from build123d import *

# Parameters (mm, degrees)
SKETCH1_W                                         = 25.4
SKETCH1_H                                         = 6
SKETCH2_R                                         = 15
BOSS_EXTRUDE1_DEPTH                               = 55.54
CUT_EXTRUDE1_DEPTH                                = 62.54
SKETCH4_W                                         = 7.0104
SKETCH4_H                                         = 61.54
F_2_CLEARANCE_HOLE1_D                             = 2.5
F_2_CLEARANCE_HOLE1_DEPTH                         = 12
SKETCH7_W                                         = 1.25
SKETCH7_H                                         = 16.341500105
CSK_FOR_8_FLAT_HEAD_MACHINE_SCREW_100_D           = 4.5
CSK_FOR_8_FLAT_HEAD_MACHINE_SCREW_100_DEPTH       = 61.54
CSK_FOR_8_FLAT_HEAD_MACHINE_SCREW_100_CSINK_D     = 9.4
CSK_FOR_8_FLAT_HEAD_MACHINE_SCREW_100_CSINK_ANGLE = 90
SKETCH11_R                                        = 10.3124
CUT_EXTRUDE2_DEPTH                                = 38.1


with BuildPart() as part:
    # Sketch1 → Revolve1 (revolve)
    with BuildSketch(Plane.XZ):
        with Locations((12.7, 58.54)):
            Rectangle(SKETCH1_W, SKETCH1_H)
    revolve(axis=Axis((0, 0, 61.54), (0, 0, -1)))

    # Sketch2 → Boss-Extrude1 (add)
    with BuildSketch(Plane(origin=(0, 0, 55.54), x_dir=(-1, 0, 0), z_dir=(0, 0, -1))):
        Circle(SKETCH2_R)
    extrude(amount=BOSS_EXTRUDE1_DEPTH)

    # Sketch3 → Cut-Extrude1 (cut, through all)
    with BuildSketch(Plane(origin=(0, 0, 0), x_dir=(-1, 0, 0), z_dir=(0, 0, -1))):
        with BuildLine():
            Line((2.5, 9.058499895), (-2.5, 9.058499895))
            Line((-2.5, 9.058499895), (-2.5, 6.538348415))
            ThreePointArc((-2.5, 6.538348415), (0, 7), (2.5, 6.538348415))
            Line((2.5, 6.538348415), (2.5, 9.058499895))
        make_face()
    extrude(amount=-CUT_EXTRUDE1_DEPTH, mode=Mode.SUBTRACT)

    # Sketch4 → Cut-Revolve1 (revolve, cut)
    with BuildSketch(Plane.XZ):
        with Locations((3.5052, 30.77)):
            Rectangle(SKETCH4_W, SKETCH4_H)
    revolve(axis=Axis((0, 0, 61.54), (0, 0, -1)), mode=Mode.SUBTRACT)

    # #2 Clearance Hole1
    with Locations(Plane(origin=(0, 0, 0), x_dir=(-1, 0, 0), z_dir=(0, 0, -1))):
        with Locations((-11.5, 0), (-5.75, -9.959292144), (5.75, -9.959292144), (11.5, 0), (5.75, 9.959292144), (-5.75, 9.959292144)):
            Hole(F_2_CLEARANCE_HOLE1_D / 2, depth=F_2_CLEARANCE_HOLE1_DEPTH)

    # Sketch7 → #2 Clearance Hole2 (revolve, cut)
    with BuildSketch(Plane(origin=(0, 9.058499895, 21.082), x_dir=(0, 0, -1), z_dir=(1, 0, 0))):
        with Locations((0.625, 8.170750053)):
            Rectangle(SKETCH7_W, SKETCH7_H)
    revolve(axis=Axis((0, 2.708499895, 21.082), (0, 1, 0)), mode=Mode.SUBTRACT)

    # CSK for #8 Flat Head Machine Screw (100)1
    with Locations(Plane.XY.offset(61.54)):
        with Locations((0, 20.4), (14.424978336, 14.424978336), (20.4, 0), (14.424978336, -14.424978336), (0, -20.4), (-14.424978336, -14.424978336), (-20.4, 0), (-14.424978336, 14.424978336)):
            CounterSinkHole(CSK_FOR_8_FLAT_HEAD_MACHINE_SCREW_100_D / 2, CSK_FOR_8_FLAT_HEAD_MACHINE_SCREW_100_CSINK_D / 2, depth=CSK_FOR_8_FLAT_HEAD_MACHINE_SCREW_100_DEPTH, counter_sink_angle=CSK_FOR_8_FLAT_HEAD_MACHINE_SCREW_100_CSINK_ANGLE)

    # Sketch11 → Cut-Extrude2 (cut)
    with BuildSketch(Plane.XY.offset(61.54)):
        Circle(SKETCH11_R)
    extrude(amount=-CUT_EXTRUDE2_DEPTH, mode=Mode.SUBTRACT)


solid = part.part
Work out the finished part from the listing and answer in its coordinate system (mm). A direction names the side the tool comes from. Give positions to 0.01 mm unless a question says otherwise; leave off trailing zeros. Loops run counter-clockwise (first coordinate to the right, second up) from the corner with the lowest first, then second, coordinate; pieces in that order, holes last. Notation, with made-up numbers: (38.25, 64.25) -> (84.25, 64.25) arc R25 ccw to (84.25, 77.25) -> close; hole circle Ø7 at (36.5, -25.75). An arc over 180 degrees is marked (long way). Use a Markdown table: item, result. Add a question column.
1. Find the intervals of material crossed by probe 1 along Y at (x, z) = (0, 38.5); probe 2 along Y at (x, z) = (-5.75, 8); probe 3 along Y at (x, z) = (0.5, 12.5), in increasing order.
2. For faces 3 (the flat face through (-6, 10, 12)), 4 (the flat face through (0, 9.058, 12)), 5 (the conical face through (-22.59, -0.91, 59.21)), determine the directions among +Z, -Z, +X, -X, +Y, -Y from which every point of the face is accessible in a straight line to the end or side of a thin tool.
3. Determine the mould class of faces 1 (the cylindrical face through (-5.506, 24.796, 58.582)), 2 (the cylindrical face through (5.54, 8.7, 42.76)) for opening direction Y: released by +Y, released by -Y, zero draft, split by the parting line, or undercut.
4. Section A-A on x = 0 is taken. State how many separate pieces and enclosed holes the cut face has, and give its area (3 significant figures).
5. Flat-ended cylindrical pins translate along their axes: pin 1 Ø12 at (y, z) = (3, 26) entering from +X; pin 2 Ø0.8 at (x, y) = (6, 10) entering from -Z; pin 3 Ø6 at (x, y) = (3, 3) entering from +Z. Find the tip coordinate at first contact, or state that the pin passes through.
6. Section B-B on x = 20.4 is taken. Determine the outline of the cut face in (y, z).
Results below:
| question | item | result |
|---|---|---|
| 1 | probe 1 | y = -15 to -10.31, 10.31 to 15 |
| 1 | probe 2 | y = -13.85 to -11.21, -8.71 to -4.01, 4.01 to 8.71, 11.21 to 13.85 |
| 1 | probe 3 | y = -14.99 to -6.99, 9.06 to 14.99 |
| 2 | face 3 | -Z |
| 2 | face 4 | +Z, -Z |
| 2 | face 5 | +Z |
| 3 | face 1 | split by the parting line |
| 3 | face 2 | undercut |
| 4 | separate pieces | 5 |
| 4 | enclosed holes | 0 |
| 4 | area | 728 mm^2 |
| 5 | pin 1 | stops at x = 15 |
| 5 | pin 2 | stops at z = 12 |
| 5 | pin 3 | stops at z = 23.44 |
| 6 | outline | (-15.13, 55.54) -> (-2.25, 55.54) -> (-2.25, 59.09) -> (-4.7, 61.54) -> (-15.13, 61.54) -> close; (2.25, 55.54) -> (15.13, 55.54) -> (15.13, 61.54) -> (4.7, 61.54) -> (2.25, 59.09) -> close |
